Input: dimensioned drawing with shaded views. Units: mm. Origin: part minimum x, y, z. A direction names the side the tool comes from. Give positions to 0.01 mm unless a question says otherwise; leave off trailing zeros. Loops run counter-clockwise (first coordinate to the right, second up) from the corner with the lowest first, then second, coordinate; pieces in that order, holes last.
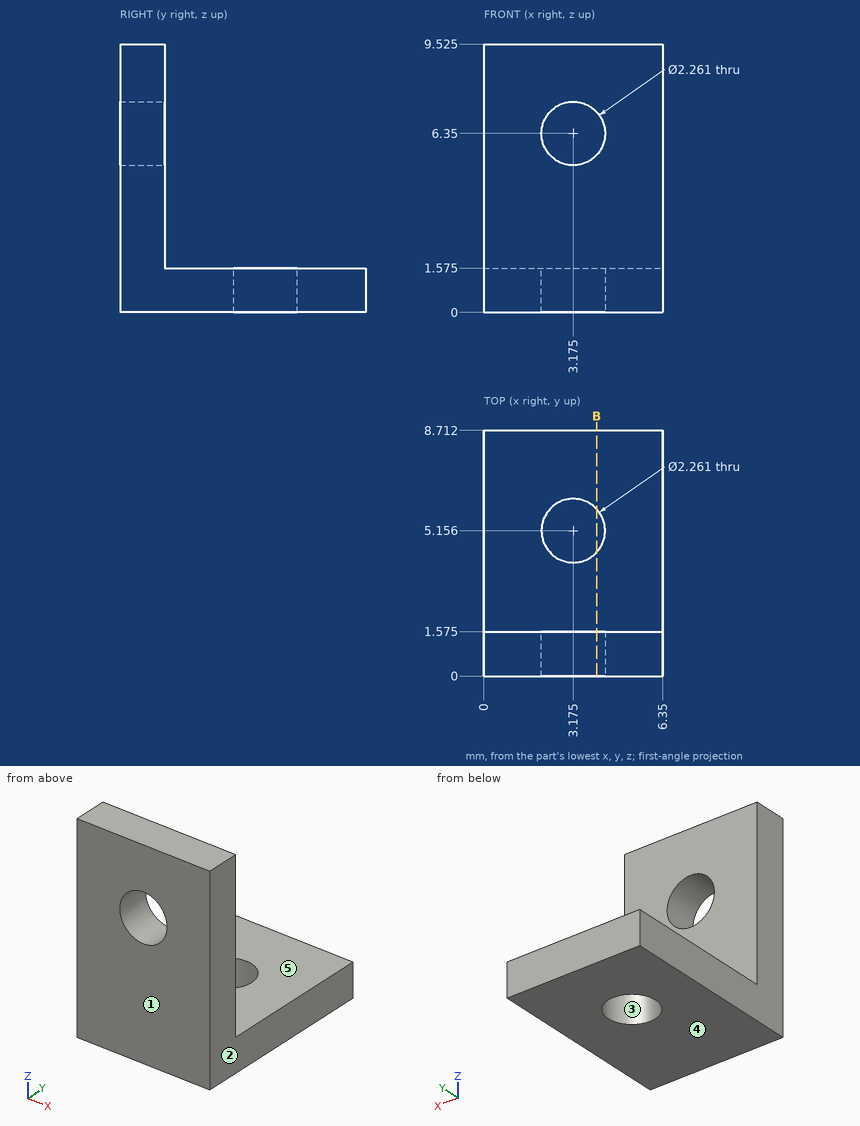
(1) First-contact query: pin 1 (2.5 mm diameter, centred on x = 3.175, z = 6.35, fed in from +Y) (1 decimal). Flat tip, straight axial feed; report the tip coordinate or a pass-through.
A:
pin 1: stops at y = 1.6
(2) Mould query, pull axis Y, two halves, no side actions, for the marked faces 1, 2 and 3. Classes: pulls with the +Y half, pulls with the -Y half, needs draft (parallel to the pull), parting line crosses it, or undercut.
A:
face 1: pulls with the -Y half
face 2: needs draft
face 3: undercut
(3) Ray query, line 1 along Y through (x, z) = (5.75, 9) (1 decimal); line 2 along X through (y, z) = (1.5, 5.5). Return the intervals inside material, ascending.
A:
line 1: y = 0 to 1.6
line 2: x = 0 to 2.43, 3.92 to 6.35
(4) Reachability of the marked faces 4 and 5 from +Z, -Z, +X, -X, +Y, -Y: full face, straight path, thin tool, end or side. Return the list, or none.
A:
face 4: -Z, +X, -X, +Y, -Y
face 5: +Z, +X, -X, +Y
(5) Section B-B, the plane x = 4. Return the cut outline in (y, z) (1 decimal).
A:
outline: (0, 0) - (4.4, 0) - (4.4, 1.6) - (1.6, 1.6) - (1.6, 5.6) - (0, 5.6) - close; (0, 7.1) - (1.6, 7.1) - (1.6, 9.5) - (0, 9.5) - close; (5.9, 0) - (8.7, 0) - (8.7, 1.6) - (5.9, 1.6) - close
